from build123d import *

# Parameters (mm, degrees)
F0_W     = 68.736359477
F0_H     = 55.0630092621
F1_DEPTH = 6.35
F2_R     = 6.34999


# Not quite as in the source:
# - a fillet or chamfer is up to 0.001 mm smaller than in the source, because OpenCascade refuses the exact size


with BuildPart() as f1:
    # F0 (on Top) → F1 (new body)
    with BuildSketch(Plane.XY):
        with Locations((-7.4506e-06, 2.0325183868)):
            Rectangle(F0_W, F0_H)
    extrude(amount=F1_DEPTH)

    # F2 (radius 6.35 in the source; OpenCascade refuses exactly that, so slightly less here)
    f2_edges = [f1.edges().sort_by_distance(p)[0] for p in [
        (-7e-06, 29.564023, 6.35),
        (34.368172, 2.032518, 6.35),
        (-34.368187, 2.032518, 6.35),
    ]]
    fillet(f2_edges, radius=F2_R)


solid = f1.part
Verification items for the finished model (mm, model axes). Give positions to 0.01 mm unless a question says otherwise; leave off trailing zeros. Write each loop counter-clockwise with the first axis right and the second up, starting at its lowest first coordinate (ties: lowest second). Pieces come first, ordered by that corner, then holes. Notation, with made-up numbers: M -24,-12.75 L -5,-12.75 A20 cw -5,18.25 Z; hole C 72.25,-21.5 d2. An arc over 180 degrees is marked long. Put each result on its own line as item: value. Start each with the question number.
1. Section check C-C (z = 5). Record the cut outline in (x, y).
2. Scan lines: line 1 along X through (y, z) = (22.5, 0.75); line 2 along X through (y, z) = (15, 4); line 3 along Y through (x, z) = (-2, 0.5). Record each from-to range of solid material in increasing order. Write a range as [from, to].
3. Go/stop test with flat-tipped pins: pin 1 Ø1 at (y, z) = (8.5, 1.5) entering from -X; pin 2 Ø1 at (x, z) = (-22.5, 2) entering from +Y. Record where each tip stops, or that it passes through.
Answer list:
1. outline: M -31.93,-25.5 L 31.93,-25.5 L 31.93,27.13 L -31.93,27.13 Z
2. line 1: [-34.32, 34.32]
2. line 2: [-32.95, 32.95]
2. line 3: [-25.5, 29.54]
3. pin 1: x = -34.29
3. pin 2: y = 29.38
